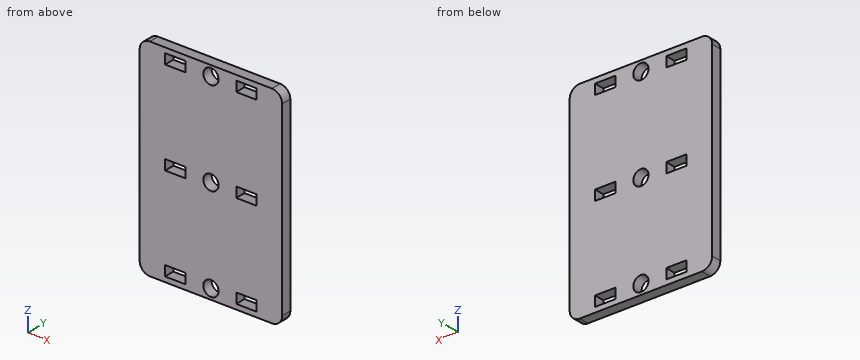
from build123d import *

# Parameters (mm, degrees)
SKETCH1_R           = 2.25
BOSS_EXTRUDE1_DEPTH = 2
FILLET1_R           = 10.25
FILLET2_R           = 2
SKETCH2_R           = 1.5
SKETCH2_W           = 4
SKETCH2_H           = 2
CUT_EXTRUDE1_DEPTH  = 2
FILLET3_R           = 8
SKETCH3_W           = 40.842978794
SKETCH3_H           = 39.737994682
CUT_EXTRUDE2_DEPTH  = 2


with BuildPart() as part:
    # Sketch1 → Boss-Extrude1 (new body)
    with BuildSketch(Plane(origin=(0, 0, 0), x_dir=(1, 0, 0), z_dir=(0, 1, 0))):
        Polygon((0, 0), (37.5, 0), (37.5, -10.25), (65.5, -10.25), (65.5, -0.75), (65.5, 21.25), (65.5, 30.75), (37.5, 30.75), (37.5, 20.5), (0, 20.5), align=None)
        with Locations(Location((10.25, 10.25, 0), (0, 0, 270))):
            Circle(SKETCH1_R, mode=Mode.SUBTRACT)
    extrude(amount=BOSS_EXTRUDE1_DEPTH)

    # Fillet1
    fillet1_edges = [part.edges().sort_by_distance(p)[0] for p in [
        (0, 1, -20.5),
        (0, 1, 0),
    ]]
    fillet(fillet1_edges, radius=FILLET1_R - 0.0001)  # a hair under: the kernel refuses the full size

    # Fillet2
    fillet2_edges = [part.edges().sort_by_distance(p)[0] for p in [
        (37.5, 1, -30.75),
        (65.5, 1, -30.75),
        (65.5, 1, 10.25),
        (37.5, 1, 10.25),
    ]]
    fillet(fillet2_edges, radius=FILLET2_R)

    # Sketch2 → Cut-Extrude1 (cut)
    with BuildSketch(Plane(origin=(0, 2, 0), x_dir=(1, 0, 0), z_dir=(0, 1, 0))):
        with Locations(Location((51.5, 28.75, 0), (0, 0, 270))):
            Circle(SKETCH2_R)
        with Locations(Location((51.5, 10.25, 0), (0, 0, 270))):
            Circle(SKETCH2_R)
        with Locations(Location((51.5, -8.25, 0), (0, 0, 270))):
            Circle(SKETCH2_R)
        with Locations((44.5, 28.75)):
            Rectangle(SKETCH2_W, SKETCH2_H)
        with Locations((58.5, 28.75)):
            Rectangle(SKETCH2_W, SKETCH2_H)
        with Locations((44.5, 10.25)):
            Rectangle(SKETCH2_W, SKETCH2_H)
        with Locations((58.5, 10.25)):
            Rectangle(SKETCH2_W, SKETCH2_H)
        with Locations((44.5, -8.25)):
            Rectangle(SKETCH2_W, SKETCH2_H)
        with Locations((58.5, -8.25)):
            Rectangle(SKETCH2_W, SKETCH2_H)
    extrude(amount=-CUT_EXTRUDE1_DEPTH, mode=Mode.SUBTRACT)

    # Fillet3
    fillet3_edges = [part.edges().sort_by_distance(p)[0] for p in [
        (37.5, 1, -20.5),
        (37.5, 1, 0),
    ]]
    fillet(fillet3_edges, radius=FILLET3_R)

    # Sketch3 → Cut-Extrude2 (cut)
    with BuildSketch(Plane(origin=(0, 2, 0), x_dir=(1, 0, 0), z_dir=(0, 1, 0))):
        with Locations((17.078510603, 8.881002659)):
            Rectangle(SKETCH3_W, SKETCH3_H)
    extrude(amount=-CUT_EXTRUDE2_DEPTH, mode=Mode.SUBTRACT)


solid = part.part
Could you check a few things on this model? Use its own coordinates, in mm. Coordinates: 2 decimals unless noted, no trailing zeros. Order: outer loops, then holes, each group sorted by start corner. A loop starts at its lowest first (then second) coordinate and runs counter-clockwise, first axis right, second up.
Q1. Suppose I cut it at C-C on y = 0.85. Give the number of separate pieces and of enclosed holes in the cut face, and give its area (3 significant figures).
Q2. Will these pins go through, and if not, where does the flat tip stop? pin 1 (0.6 mm diameter, centred on y = 1, z = -29, fed in from -X); pin 2 (2.5 mm diameter, centred on x = 51.5, z = -28.75, fed in from -Y).
Q3. Suppose I cut it at A-A on x = 59.25. Please give me the cut outline in (y, z), and give its area (3 significant figures).
Q4. Suppose I cut it at B-B on z = -10.25. Please give me the cut outline in (x, y), and give its area (3 significant figures).
Q5. Please list where these lines run through material, in increasing order: L1, parallel to Z at x = 45.25, y = 0.9; L2, parallel to X at y = 1.55, z = 8.25; L3, parallel to Z at x = 52.5, y = 0.9.
Answer:
1. separate pieces: 1
1. enclosed holes: 9
1. area: 1,080 mm2
2. pin 1: stops at x = 37.5
2. pin 2: passes through
3. outline: (0, -30.75) - (2, -30.75) - (2, -29.75) - (0, -29.75) - close; (0, -27.75) - (2, -27.75) - (2, -11.25) - (0, -11.25) - close; (0, -9.25) - (2, -9.25) - (2, 7.25) - (0, 7.25) - close; (0, 9.25) - (2, 9.25) - (2, 10.25) - (0, 10.25) - close
3. area: 70.0 mm2
4. outline: (37.5, 0) - (42.5, 0) - (42.5, 2) - (37.5, 2) - close; (46.5, 0) - (50, 0) - (50, 2) - (46.5, 2) - close; (53, 0) - (56.5, 0) - (56.5, 2) - (53, 2) - close; (60.5, 0) - (65.5, 0) - (65.5, 2) - (60.5, 2) - close
4. area: 34.0 mm2
5. L1: z = -30.75 to -29.75, -27.75 to -11.25, -9.25 to 7.25, 9.25 to 10.25
5. L2: x = 37.5 to 42.5, 46.5 to 50, 53 to 56.5, 60.5 to 65.5
5. L3: z = -30.75 to -29.87, -27.63 to -11.37, -9.13 to 7.13, 9.37 to 10.25
